```python
from build123d import *

# Parameters (mm, degrees)
F0_R     = 1.5875
F1_DEPTH = 25.4
F2_DEPTH = 21.59


with BuildPart() as f1:
    # F0 (on Front) → F1 (new body)
    with BuildSketch(Plane.XZ):
        with BuildLine():
            ThreePointArc((-45.8923771413, 104.7758257242), (-39.2384052999, 107.6092963617), (-36.4927939024, 114.3))
            ThreePointArc((-36.4927939024, 114.3), (-46.0177939024, 123.825), (-55.5427939024, 114.3))
            ThreePointArc((-55.5427939024, 114.3), (-52.7084975407, 107.5206113974), (-45.8923771413, 104.7758257242))
        make_face()
        with BuildLine():
            ThreePointArc((-42.8427939024, 114.3), (-43.7579977016, 112.0697654539), (-45.9759883154, 111.1252752414))
            ThreePointArc((-45.9759883154, 111.1252752414), (-48.2775901033, 116.5302345461), (-42.8427939024, 114.3))
        make_face(mode=Mode.SUBTRACT)
        with BuildLine():
            Line((-29.6299272337, 65.7206308807), (-36.4927939024, 114.3))
            ThreePointArc((-36.4927939024, 114.3), (-39.2384052999, 107.6092963617), (-45.8923771413, 104.7758257242))
            Line((-45.8923771413, 104.7758257242), (-45.5578744539, 79.373623793))
            ThreePointArc((-45.5578744539, 79.373623793), (-35.0173298688, 75.5530240484), (-29.6299272337, 65.7206308807))
        make_face()
        with BuildLine():
            ThreePointArc((-45.8923771413, 104.7758257242), (-52.7084975407, 107.5206113974), (-55.5427939024, 114.3))
            Line((-55.5427939024, 114.3), (-61.1219506134, 65.2957762162))
            ThreePointArc((-61.1219506134, 65.2957762162), (-55.9979584138, 75.2733614931), (-45.5578744539, 79.373623793))
            Line((-45.5578744539, 79.373623793), (-45.8923771413, 104.7758257242))
        make_face()
        with Locations((-48.6637000366, 100.0252)):
            Circle(F0_R, mode=Mode.SUBTRACT)
        with BuildLine():
            ThreePointArc((-29.4738465188, 63.5), (-29.5129147708, 64.6130546592), (-29.6299272337, 65.7206308807))
            ThreePointArc((-29.6299272337, 65.7206308807), (-35.0173298688, 75.5530240484), (-45.5578744539, 79.373623793))
            Line((-45.5578744539, 79.373623793), (-45.3906521058, 66.6747247586))
            ThreePointArc((-45.3906521058, 66.6747247586), (-43.1186119727, 65.7597962009), (-42.1738465188, 63.5))
            ThreePointArc((-42.1738465188, 63.5), (-43.087950392, 61.2708805092), (-45.3039086946, 60.3253180329))
            Line((-45.3039086946, 60.3253180329), (-45.124157398, 47.6265901647))
            ThreePointArc((-45.124157398, 47.6265901647), (-34.8536449701, 51.5892330451), (-29.6299272337, 61.2793691193))
            ThreePointArc((-29.6299272337, 61.2793691193), (-29.5129147708, 62.3869453408), (-29.4738465188, 63.5))
        make_face()
        with BuildLine():
            ThreePointArc((-45.5578744539, 79.373623793), (-55.9979584138, 75.2733614931), (-61.1219506134, 65.2957762162))
            ThreePointArc((-61.1219506134, 65.2957762162), (-61.2238389716, 63.4845202884), (-61.1184184978, 61.6734665075))
            ThreePointArc((-61.1184184978, 61.6734665075), (-55.8245101978, 51.5720456287), (-45.124157398, 47.6265901647))
            Line((-45.124157398, 47.6265901647), (-45.3039086946, 60.3253180329))
            ThreePointArc((-45.3039086946, 60.3253180329), (-48.5235502679, 63.4566282891), (-45.3906521058, 66.6747247586))
            Line((-45.3906521058, 66.6747247586), (-45.5578744539, 79.373623793))
        make_face()
        with BuildLine():
            ThreePointArc((-45.124157398, 47.6265901647), (-55.8245101978, 51.5720456287), (-61.1184184978, 61.6734665075))
            Line((-61.1184184978, 61.6734665075), (-53.975, 0))
            ThreePointArc((-53.975, 0), (-51.2326883802, 6.6873584723), (-44.5848134725, 9.5240459012))
            Line((-44.5848134725, 9.5240459012), (-45.124157398, 47.6265901647))
        make_face()
        with BuildLine():
            Line((-33.3890422301, 17.4858067619), (-29.6299272337, 61.2793691193))
            ThreePointArc((-29.6299272337, 61.2793691193), (-34.8536449701, 51.5892330451), (-45.124157398, 47.6265901647))
            Line((-45.124157398, 47.6265901647), (-44.5848134725, 9.5240459012))
            ThreePointArc((-44.5848134725, 9.5240459012), (-37.7626415277, 6.7826883802), (-34.925, 0))
            Line((-34.925, 0), (-7.9375, 0))
            ThreePointArc((-7.9375, 0), (-5.6126600757, 5.6126600757), (0, 7.9375))
            Line((0, 7.9375), (-25.7528172131, 8.8607889455))
            ThreePointArc((-25.7528172131, 8.8607889455), (-31.4204494391, 11.5358115277), (-33.3890422301, 17.4858067619))
        make_face()
        with BuildLine():
            ThreePointArc((-44.5848134725, 9.5240459012), (-51.2326883802, 6.6873584723), (-53.975, 0))
            ThreePointArc((-53.975, 0), (-51.0634341324, -6.8547876682), (-44.1087293489, -9.5188843539))
            ThreePointArc((-44.1087293489, -9.5188843539), (-37.5952123318, -6.6134341324), (-34.925, 0))
            Line((-34.925, 0), (-41.275, 0))
            ThreePointArc((-41.275, 0), (-46.6791194908, -2.2608961267), (-44.4949378242, 3.1746819671))
            Line((-44.4949378242, 3.1746819671), (-44.5848134725, 9.5240459012))
        make_face()
        with BuildLine():
            ThreePointArc((-34.925, 0), (-37.5952123318, -6.6134341324), (-44.1087293489, -9.5188843539))
            Line((-44.1087293489, -9.5188843539), (0, -7.9375))
            ThreePointArc((0, -7.9375), (-5.6126600757, -5.6126600757), (-7.9375, 0))
            Line((-7.9375, 0), (-34.925, 0))
        make_face()
        with BuildLine():
            ThreePointArc((-7.9375, 0), (-5.6126600757, -5.6126600757), (0, -7.9375))
            ThreePointArc((0, -7.9375), (5.6126600757, -5.6126600757), (7.9375, 0))
            ThreePointArc((7.9375, 0), (5.6126600757, 5.6126600757), (0, 7.9375))
            ThreePointArc((0, 7.9375), (-5.6126600757, 5.6126600757), (-7.9375, 0))
        make_face()
        with BuildLine():
            ThreePointArc((3.175, 0), (0, -3.175), (-3.175, 0))
            ThreePointArc((-3.175, 0), (0, 3.175), (3.175, 0))
        make_face(mode=Mode.SUBTRACT)
    extrude(amount=F1_DEPTH)

    # F0 (on Front) → F2 (join)
    with BuildSketch(Plane.XZ):
        with BuildLine():
            ThreePointArc((-45.8923771413, 104.7758257242), (-39.2384052999, 107.6092963617), (-36.4927939024, 114.3))
            ThreePointArc((-36.4927939024, 114.3), (-46.0177939024, 123.825), (-55.5427939024, 114.3))
            ThreePointArc((-55.5427939024, 114.3), (-52.7084975407, 107.5206113974), (-45.8923771413, 104.7758257242))
        make_face()
        with BuildLine():
            ThreePointArc((-42.8427939024, 114.3), (-43.7579977016, 112.0697654539), (-45.9759883154, 111.1252752414))
            ThreePointArc((-45.9759883154, 111.1252752414), (-48.2775901033, 116.5302345461), (-42.8427939024, 114.3))
        make_face(mode=Mode.SUBTRACT)
        with BuildLine():
            Line((-29.6299272337, 65.7206308807), (-36.4927939024, 114.3))
            ThreePointArc((-36.4927939024, 114.3), (-39.2384052999, 107.6092963617), (-45.8923771413, 104.7758257242))
            Line((-45.8923771413, 104.7758257242), (-45.5578744539, 79.373623793))
            ThreePointArc((-45.5578744539, 79.373623793), (-35.0173298688, 75.5530240484), (-29.6299272337, 65.7206308807))
        make_face()
        with BuildLine():
            ThreePointArc((-45.8923771413, 104.7758257242), (-52.7084975407, 107.5206113974), (-55.5427939024, 114.3))
            Line((-55.5427939024, 114.3), (-61.1219506134, 65.2957762162))
            ThreePointArc((-61.1219506134, 65.2957762162), (-55.9979584138, 75.2733614931), (-45.5578744539, 79.373623793))
            Line((-45.5578744539, 79.373623793), (-45.8923771413, 104.7758257242))
        make_face()
        with Locations((-48.6637000366, 100.0252)):
            Circle(F0_R, mode=Mode.SUBTRACT)
        with BuildLine():
            ThreePointArc((-29.4738465188, 63.5), (-29.5129147708, 64.6130546592), (-29.6299272337, 65.7206308807))
            ThreePointArc((-29.6299272337, 65.7206308807), (-35.0173298688, 75.5530240484), (-45.5578744539, 79.373623793))
            Line((-45.5578744539, 79.373623793), (-45.3906521058, 66.6747247586))
            ThreePointArc((-45.3906521058, 66.6747247586), (-43.1186119727, 65.7597962009), (-42.1738465188, 63.5))
            ThreePointArc((-42.1738465188, 63.5), (-43.087950392, 61.2708805092), (-45.3039086946, 60.3253180329))
            Line((-45.3039086946, 60.3253180329), (-45.124157398, 47.6265901647))
            ThreePointArc((-45.124157398, 47.6265901647), (-34.8536449701, 51.5892330451), (-29.6299272337, 61.2793691193))
            ThreePointArc((-29.6299272337, 61.2793691193), (-29.5129147708, 62.3869453408), (-29.4738465188, 63.5))
        make_face()
        with BuildLine():
            ThreePointArc((-45.5578744539, 79.373623793), (-55.9979584138, 75.2733614931), (-61.1219506134, 65.2957762162))
            ThreePointArc((-61.1219506134, 65.2957762162), (-61.2238389716, 63.4845202884), (-61.1184184978, 61.6734665075))
            ThreePointArc((-61.1184184978, 61.6734665075), (-55.8245101978, 51.5720456287), (-45.124157398, 47.6265901647))
            Line((-45.124157398, 47.6265901647), (-45.3039086946, 60.3253180329))
            ThreePointArc((-45.3039086946, 60.3253180329), (-48.5235502679, 63.4566282891), (-45.3906521058, 66.6747247586))
            Line((-45.3906521058, 66.6747247586), (-45.5578744539, 79.373623793))
        make_face()
        with BuildLine():
            ThreePointArc((-45.124157398, 47.6265901647), (-55.8245101978, 51.5720456287), (-61.1184184978, 61.6734665075))
            Line((-61.1184184978, 61.6734665075), (-53.975, 0))
            ThreePointArc((-53.975, 0), (-51.2326883802, 6.6873584723), (-44.5848134725, 9.5240459012))
            Line((-44.5848134725, 9.5240459012), (-45.124157398, 47.6265901647))
        make_face()
        with BuildLine():
            Line((-33.3890422301, 17.4858067619), (-29.6299272337, 61.2793691193))
            ThreePointArc((-29.6299272337, 61.2793691193), (-34.8536449701, 51.5892330451), (-45.124157398, 47.6265901647))
            Line((-45.124157398, 47.6265901647), (-44.5848134725, 9.5240459012))
            ThreePointArc((-44.5848134725, 9.5240459012), (-37.7626415277, 6.7826883802), (-34.925, 0))
            Line((-34.925, 0), (-7.9375, 0))
            ThreePointArc((-7.9375, 0), (-5.6126600757, 5.6126600757), (0, 7.9375))
            Line((0, 7.9375), (-25.7528172131, 8.8607889455))
            ThreePointArc((-25.7528172131, 8.8607889455), (-31.4204494391, 11.5358115277), (-33.3890422301, 17.4858067619))
        make_face()
        with BuildLine():
            ThreePointArc((-44.5848134725, 9.5240459012), (-51.2326883802, 6.6873584723), (-53.975, 0))
            ThreePointArc((-53.975, 0), (-51.0634341324, -6.8547876682), (-44.1087293489, -9.5188843539))
            ThreePointArc((-44.1087293489, -9.5188843539), (-37.5952123318, -6.6134341324), (-34.925, 0))
            Line((-34.925, 0), (-41.275, 0))
            ThreePointArc((-41.275, 0), (-46.6791194908, -2.2608961267), (-44.4949378242, 3.1746819671))
            Line((-44.4949378242, 3.1746819671), (-44.5848134725, 9.5240459012))
        make_face()
        with BuildLine():
            ThreePointArc((-34.925, 0), (-37.5952123318, -6.6134341324), (-44.1087293489, -9.5188843539))
            Line((-44.1087293489, -9.5188843539), (0, -7.9375))
            ThreePointArc((0, -7.9375), (-5.6126600757, -5.6126600757), (-7.9375, 0))
            Line((-7.9375, 0), (-34.925, 0))
        make_face()
        with BuildLine():
            ThreePointArc((-7.9375, 0), (-5.6126600757, -5.6126600757), (0, -7.9375))
            ThreePointArc((0, -7.9375), (5.6126600757, -5.6126600757), (7.9375, 0))
            ThreePointArc((7.9375, 0), (5.6126600757, 5.6126600757), (0, 7.9375))
            ThreePointArc((0, 7.9375), (-5.6126600757, 5.6126600757), (-7.9375, 0))
        make_face()
        with BuildLine():
            ThreePointArc((3.175, 0), (0, -3.175), (-3.175, 0))
            ThreePointArc((-3.175, 0), (0, 3.175), (3.175, 0))
        make_face(mode=Mode.SUBTRACT)
        with BuildLine():
            ThreePointArc((-34.925, 0), (-37.7626415277, 6.7826883802), (-44.5848134725, 9.5240459012))
            Line((-44.5848134725, 9.5240459012), (-44.4949378242, 3.1746819671))
            ThreePointArc((-44.4949378242, 3.1746819671), (-42.2208805092, 2.2608961267), (-41.275, 0))
            Line((-41.275, 0), (-34.925, 0))
        make_face()
    extrude(amount=F2_DEPTH)


solid = f1.part
```
Source: CAD feature listing. Evaluate the final solid. Frame: model axes, mm. A direction names the side the tool comes from. Round coordinates to 2 decimals unless told otherwise and drop trailing zeros. Write each loop counter-clockwise with the first axis right and the second up, starting at its lowest first coordinate (ties: lowest second). Pieces come first, ordered by that corner, then holes. Notation, with made-up numbers: M 79,88.5 L 98,88.5 A24 ccw 98,110.5 Z; hole C 32,75 d7. An arc over 180 degrees is marked long. Answer as a JSON object with one key per item and string values. Group by question number.
(1) Section query D-D on z = 19.5. Output: boundary loops of the cut face in (x, y), then the cut area to 3 significant figures.
(2) Section query A-A on x = -31.5. Output: boundary loops of the cut face in (y, z), then the cut area to 3 significant figures.
(3) Ray query, line 1 (Z direction, x = -44.45, y = -6.25) (3 decimals); line 2 (X direction, y = -9, z = 114.3); line 3 (Z direction, x = -46, y = -18). Return the intervals inside material, ascending. Write a range as [from, to].
(4) Section query C-C on z = 4.5. Output: boundary loops of the cut face in (x, y).
(5) Mould query, pull axis X, two halves, no side actions, for faces 3 (the cylindrical face through (-45.808, -12.522, 123.823)), 4 (the cylindrical face through (-3.03, -12.52, 0.95)), 5 (the flat face through (-40, -21.59, 5)), 6 (the flat face through (-31.536, -12.522, 39.076)). Classes: +X half, -X half, draft (parallel to the pull), parting line (faces both ways), or undercut.
(6) Reachability of faces 1 (the cylindrical face through (-61.224, -12.522, 63.51)), 2 (the flat face through (-38, -23, 0)) from +Z, -Z, +X, -X, +Y, -Y: full face, straight path, thin tool, end or side. Return the list, or none.
(7) Section query B-B on y = -3.5. State how many separate pieces and enclosed holes the cut face has, then the cut area to 3 significant figures.
(8) First-contact query: pin 1 (4 mm diameter, centred on x = -14.5, y = -7.5, fed in from -Z); pin 2 (4 mm diameter, centred on y = -10, z = 78, fed in from +X); pin 3 (5 mm diameter, centred on y = -19.5, z = 27.5, fed in from -X); pin 4 (2.5 mm diameter, centred on x = -48.66, z = 100.03, fed in from -Y). Flat tips, straight axial feed; report the tip coordinate or a pass-through.
Computed values:
{
 "1": {"outline": "M -56.23,-25.4 L -33.22,-25.4 L -33.22,0 L -56.23,0 Z", "area": "585 mm^2"},
 "2": {"outline": "M -25.4,-9.07 L 0,-9.07 L 0,11.63 L -25.4,11.63 Z; M -25.4,39.49 L 0,39.49 L 0,78.96 L -25.4,78.96 Z", "area": "1,530 mm^2"},
 "3": {"line 1": "[-9.525, -3.175], [3.175, 60.455], [66.545, 111.539], [117.061, 123.695]", "line 2": "[-55.54, -49.19], [-42.84, -36.49]", "line 3": "[-9.4, -2.77], [2.77, 60.39], [66.61, 111.13], [117.47, 123.82]"},
 "4": {"outline": "M -54.5,-25.4 L -44.51,-25.4 L -44.51,-21.59 L -36.06,-21.59 L -36.06,-25.4 L 6.54,-25.4 L 6.54,0 L -54.5,0 Z"},
 "5": {"face 3": "parting line", "face 4": "undercut", "face 5": "undercut", "face 6": "+X half"},
 "6": {"face 1": "-X, +Y, -Y", "face 2": "-Y"},
 "7": {"separate pieces": "1", "enclosed holes": "5", "area": "3,790 mm^2"},
 "8": {"pin 1": "z = -8.53", "pin 2": "x = -31.08", "pin 3": "x = -57.45", "pin 4": "through"}
}
